Check sheet for the modelled part. Datum: model origin and axes. Units: mm. Round coordinates to 2 decimals unless told otherwise and drop trailing zeros. Loops run counter-clockwise (first coordinate to the right, second up) from the corner with the lowest first, then second, coordinate; pieces in that order, holes last. Notation, with made-up numbers: M 38,18 L 57,18 A16 cw 57,47 Z; hole C 55.25,-25 d5. An arc over 180 degrees is marked long. One line per question, with ' | ' between items. Start each with the question number.
(1) Section check B-B (x = 14). Record the boundary of the cut face in (y, z).
(2) Section check D-D (z = 18). Record the boundary of the cut face in (x, y), and give its area (3 significant figures).
(3) Section check C-C (y = -1.9). Count the separate pieces of the cut face and the enclosed holes in it, and give its area (3 significant figures).
(4) Section check A-A (z = -8.5). Record the boundary of the cut face in (x, y), and give its area (3 significant figures).
(5) Go/stop test with a flat-tipped pin: P1, Ø5, axis at x = 23.25, z = 0, coming from the +Y side. Record where the tip stops, or that it passes through.
(6) Thickness scan on probe 1 along Z at (x, y) = (18, -1.9); probe 2 along Z at (x, y) = (0, -1.95); probe 3 along Z at (x, y) = (-6.5, -2.1). Record the ranges inside material, lowest first. Write a range as [from, to].
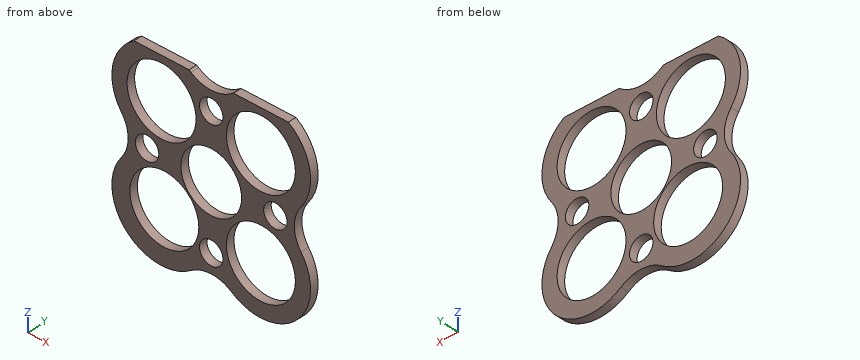
```python
from build123d import *

# Parameters (mm, degrees)
F0_R     = 12.5
F0_R_2   = 4.25
F0_R_3   = 11
F1_DEPTH = 3


with BuildPart() as f1:
    # F0 (on Front) → F1 (new body)
    with BuildSketch(Plane.XZ):
        with BuildLine():
            ThreePointArc((32.531102, -7.377049), (30.122145, 0), (32.531102, 7.377049))
            ThreePointArc((32.531102, 7.377049), (35.719014, 21.168052), (27.949874, 33))
            Line((27.949874, 33), (8.050126, 33))
            ThreePointArc((8.050126, 33), (7.710916, 32.769386), (7.377049, 32.531102))
            ThreePointArc((7.377049, 32.531102), (0, 30.122145), (-7.377049, 32.531102))
            ThreePointArc((-7.377049, 32.531102), (-7.710916, 32.769386), (-8.050126, 33))
            Line((-8.050126, 33), (-27.949874, 33))
            ThreePointArc((-27.949874, 33), (-35.719014, 21.168052), (-32.531102, 7.377049))
            ThreePointArc((-32.531102, 7.377049), (-30.122145, 0), (-32.531102, -7.377049))
            ThreePointArc((-32.531102, -7.377049), (-30.727922, -30.727922), (-7.377049, -32.531102))
            ThreePointArc((-7.377049, -32.531102), (0, -30.122145), (7.377049, -32.531102))
            ThreePointArc((7.377049, -32.531102), (30.727922, -30.727922), (32.531102, -7.377049))
        make_face()
        with Locations((-17, -17)):
            Circle(F0_R, mode=Mode.SUBTRACT)
        with Locations((0, -23.25)):
            Circle(F0_R_2, mode=Mode.SUBTRACT)
        with Locations((18, -18)):
            Circle(F0_R, mode=Mode.SUBTRACT)
        with Locations((-23.25, 0)):
            Circle(F0_R_2, mode=Mode.SUBTRACT)
        with Locations((-18, 18)):
            Circle(F0_R, mode=Mode.SUBTRACT)
        Circle(F0_R_3, mode=Mode.SUBTRACT)
        with Locations((23.25, 0)):
            Circle(F0_R_2, mode=Mode.SUBTRACT)
        with Locations((0, 23.25)):
            Circle(F0_R_2, mode=Mode.SUBTRACT)
        with Locations((18, 18)):
            Circle(F0_R, mode=Mode.SUBTRACT)
    extrude(amount=F1_DEPTH)


solid = f1.part
```
The answers:
1) outline: M -3,-35.55 L 0,-35.55 L 0,-29.84 L -3,-29.84 Z; M -3,-6.16 L 0,-6.16 L 0,6.16 L -3,6.16 Z; M -3,29.84 L 0,29.84 L 0,33 L -3,33 Z
2) outline: M -36,-3 L -30.5,-3 L -30.5,0 L -36,0 Z; M -5.5,-3 L 5.5,-3 L 5.5,0 L -5.5,0 Z; M 30.5,-3 L 36,-3 L 36,0 L 30.5,0 Z | area: 66.0 mm²
3) separate pieces: 1 | enclosed holes: 9 | area: 1,860 mm²
4) outline: M -33.29,-3 L -26.17,-3 L -26.17,0 L -33.29,0 Z; M -7.83,-3 L -6.98,-3 L -6.98,0 L -7.83,0 Z; M 6.98,-3 L 9.88,-3 L 9.88,0 L 6.98,0 Z; M 26.12,-3 L 33.29,-3 L 33.29,0 L 26.12,0 Z | area: 54.1 mm²
5) P1: through
6) probe 1: [-36, -30.5], [-5.5, 5.5], [30.5, 33] | probe 2: [-30.12, -27.5], [-19, -11], [11, 19], [27.5, 30.12] | probe 3: [-31.95, -23.78], [-10.22, -8.87], [8.87, 13.1], [22.9, 31.95]
